Source: CAD feature listing. Evaluate the final solid. Frame: model axes, mm. Face numbers are marked on the shaded views. Give positions to 0.01 mm unless a question says otherwise; leave off trailing zeros. Order: outer loops, then holes, each group sorted by start corner. A loop starts at its lowest first (then second) coordinate and runs counter-clockwise, first axis right, second up. Notation, with made-up numbers: (73.25, -33) -> (132.25, -33) arc R21 ccw to (132.25, -1) -> close; hole circle Ø8 at (46, 14.5). An arc over 180 degrees is marked (long way). Use CSV: the item, a comma, the result in double quotes.
Autodesk Inventor part; units mm, degrees
ref_plane "YZ Plane" through (0, 0, 0) normal (1, 0, 0) x (0, 1, 0)
ref_plane "XZ Plane" through (0, 0, 0) normal (0, 1, 0) x (-1, 0, 0)
ref_plane "XY Plane" through (0, 0, 0) normal (0, 0, 1) x (1, 0, 0)
ref_plane "Work Plane1" through (0, 0, 0) normal (0, 0, 1) x (1, 0, 0)
sketch "Sketch1" plane through (0, 0, 0) normal (0, 0, 1) x (1, 0, 0)
  circle A0 centre (-53.7689, -11.7651) radius 3.2332
  circle A1 centre (-53.7689, -11.7651) radius 4.05
  circle A2 centre (-53.7689, -11.7651) radius 6.5
  point P0 (0, 0)
  point P1 (-52.2586, -9.305)
  dimension "d0" = 8.1
  dimension "d1" = 13
extrude "Extrusion1" add sketch "Sketch1" along normal blind 20 contours A0 | A1 | A2
chamfer "Chamfer1" distance 0.5 angle 45 2 edges at (-60.2689, -11.7651, 0) (-60.2689, -11.7651, 20)
sketch "Sketch2" plane through (-53.7689, -11.7651, 20) normal (0, 0, 1) x (1, 0, 0)
  circle A0 centre (0, 0) radius 4.05
  point P0 (53.7689, 11.7651)
  dimension "d7" = 8.1
extrude "Extrusion2" cut sketch "Sketch2" against normal blind 20
properties part number "Spacers"
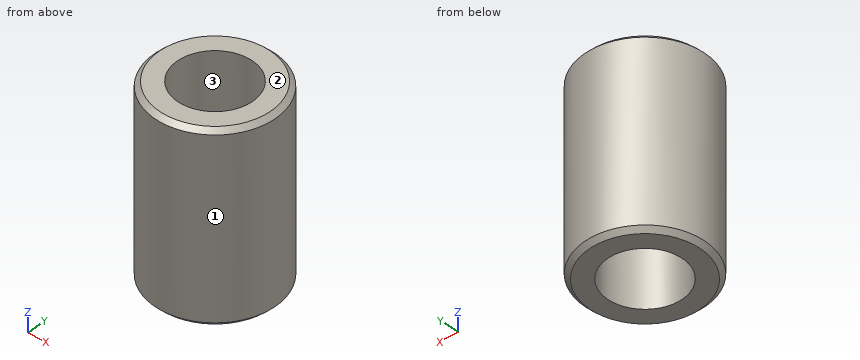
1. Section query A-A on z = 5. Return loops of the section in (x, y), plus the area to 3 significant figures.
Answer below:
outline,"circle Ø13 at (-53.77, -11.77); hole circle Ø8.1 at (-53.77, -11.77)"
area,"81.2 mm²"
2. Mould query, pull axis X, two halves, no side actions, for the marked faces 1, 2 and 3. Classes: released by +X, released by -X, zero draft, split by the parting line, or undercut.
Answer below:
face 1,"split by the parting line"
face 2,"zero draft"
face 3,"undercut"
3. Ray query, line 1 along X through (y, z) = (-12, 12); line 2 along Y through (x, z) = (-55, 10); line 3 along Y through (x, z) = (-55.5, 7.5). Return the intervals inside material, ascending.
Answer below:
line 1,"x = -60.26 to -57.81, -49.73 to -47.27"
line 2,"y = -18.15 to -15.62, -7.91 to -5.38"
line 3,"y = -18.03 to -15.43, -8.1 to -5.5"
4. Pin query (flat end, axial travel): P1, Ø6, axis at x = -59, z = 5, coming from the +Y side; P2, Ø1, axis at x = -56, z = 5, coming from the -Y side; P3, Ø1.5, axis at x = -51.5, z = 8, coming from the -Y side. Return the tip coordinate at first contact, or that it passes through.
Answer below:
P1,"stops at y = -5.66"
P2,"stops at y = -18.03"
P3,"stops at y = -18.09"
